Source: CAD feature listing. Evaluate the final solid. Frame: model axes, mm. A direction names the side the tool comes from. Give positions to 0.01 mm unless a question says otherwise; leave off trailing zeros. Loops run counter-clockwise (first coordinate to the right, second up) from the corner with the lowest first, then second, coordinate; pieces in that order, holes last.
```python
from build123d import *

# Parameters (mm, degrees)
SKETCH1_R               = 6.35
BOSS_EXTRUDE1_DEPTH     = 50.8
SKETCH2_W               = 82.55
SKETCH2_H               = 66.675
CUT_EXTRUDE1_DEPTH      = 20.05
CUT_EXTRUDE1_DEPTH_BACK = 20.05
FILLET1_R               = 6.35
FILLET2_R               = 9.525
FILLET3_R               = 9.525
FILLET4_R               = 9.525


with BuildPart() as part:
    # Sketch1 → Boss-Extrude1 (new body, symmetric)
    with BuildSketch(Plane(origin=(0, 0, 0), x_dir=(0, 0, -1), z_dir=(1, 0, 0))):
        with BuildLine():
            Line((9.525, 36.5125), (14.473290811, 46.0375))
            Line((14.473290811, 46.0375), (-9.525, 46.0375))
            Line((-9.525, 46.0375), (-9.525, 36.5125))
            Line((-9.525, 36.5125), (-9.525, 16.497783942))
            ThreePointArc((-9.525, 16.497783942), (-19.05, 0), (-9.525, -16.497783942))
            Line((-9.525, -16.497783942), (-9.525, -36.5125))
            Line((-9.525, -36.5125), (-14.473290811, -46.0375))
            Line((-14.473290811, -46.0375), (9.525, -46.0375))
            Line((9.525, -46.0375), (9.525, -36.5125))
            Line((9.525, -36.5125), (9.525, -16.497783942))
            ThreePointArc((9.525, -16.497783942), (19.05, 0), (9.525, 16.497783942))
            Line((9.525, 16.497783942), (9.525, 36.5125))
        make_face()
        Circle(SKETCH1_R, mode=Mode.SUBTRACT)
    extrude(amount=BOSS_EXTRUDE1_DEPTH, both=True)

    # Sketch2 → Cut-Extrude1 (cut, two sides)
    with BuildSketch(Plane.XY) as cut_extrude1_sk:
        Rectangle(SKETCH2_W, SKETCH2_H)
    extrude(amount=CUT_EXTRUDE1_DEPTH, mode=Mode.SUBTRACT)
    extrude(cut_extrude1_sk.sketch, amount=-CUT_EXTRUDE1_DEPTH_BACK, mode=Mode.SUBTRACT)

    # Fillet1
    fillet1_edges = [part.edges().sort_by_distance(p)[0] for p in [
        (-41.275, 33.3375, 0),
        (41.275, -33.3375, 0),
        (41.275, 33.3375, 0),
        (-41.275, -33.3375, 0),
    ]]
    fillet(fillet1_edges, radius=FILLET1_R)

    # Fillet2
    fillet2_edges = [part.edges().sort_by_distance(p)[0] for p in [
        (46.0375, 16.497783942, -9.525),
        (46.0375, -16.497783942, -9.525),
        (46.0375, -16.497783942, 9.525),
        (46.0375, 16.497783942, 9.525),
        (-46.0375, 16.497783942, -9.525),
        (-46.0375, -16.497783942, -9.525),
        (-46.0375, -16.497783942, 9.525),
        (-46.0375, 16.497783942, 9.525),
    ]]
    fillet(fillet2_edges, radius=FILLET2_R)

    # Fillet3
    fillet3_edges = [part.edges().sort_by_distance(p)[0] for p in [
        (0, -46.0375, -9.525),
        (0, 46.0375, 9.525),
    ]]
    fillet(fillet3_edges, radius=FILLET3_R)

    # Fillet4
    fillet4_edges = [part.edges().sort_by_distance(p)[0] for p in [
        (0, -36.5125, 9.525),
        (0, 36.5125, -9.525),
    ]]
    fillet(fillet4_edges, radius=FILLET4_R)


solid = part.part
```
(1) Ray query, line 1 along X through (y, z) = (6.5, 5) (3 decimals); line 2 along Z through (x, y) = (45, 0); line 3 along Z through (x, y) = (43, 23) (3 decimals). Return the intervals inside material, ascending.
A:
line 1: x = -50.8 to -41.275, 41.275 to 50.8
line 2: z = -19.05 to -6.35, 6.35 to 19.05
line 3: z = -9.525 to 9.525
(2) Section A-A, the plane y = 0. Return the cut outline in (x, z) (3 decimals).
A:
outline: (-50.8, -19.05) - (-41.275, -19.05) - (-41.275, -6.35) - (-50.8, -6.35) - close; (-50.8, 6.35) - (-41.275, 6.35) - (-41.275, 19.05) - (-50.8, 19.05) - close; (41.275, -19.05) - (50.8, -19.05) - (50.8, -6.35) - (41.275, -6.35) - close; (41.275, 6.35) - (50.8, 6.35) - (50.8, 19.05) - (41.275, 19.05) - close
(3) Section D-D, the plane y = -12.5. Return the cut outline in (x, z) (3 decimals), then the cut area to 3 significant figures.
A:
outline: (-50.8, -14.375) - (-41.275, -14.375) - (-41.275, 14.375) - (-50.8, 14.375) - close; (41.275, -14.375) - (50.8, -14.375) - (50.8, 14.375) - (41.275, 14.375) - close
area: 548 mm2
(4) First-contact query: pin 1 (9.5 mm diameter, centred on x = -12, z = 4.5, fed in from +Y); pin 2 (14 mm diameter, centred on x = 23.5, y = 31, fed in from -Z); pin 3 (2 mm diameter, centred on x = 18.5, y = 33.5, fed in from +Z) (3 decimals); pin 4 (12 mm diameter, centred on x = -23, y = -28, fed in from -Z) (3 decimals). Flat tips, straight axial feed; report the tip coordinate or a pass-through.
A:
pin 1: stops at y = 46.04
pin 2: stops at z = -10.32
pin 3: stops at z = 9.525
pin 4: stops at z = -9.525
(5) Reachability of faces 1 (the flat face through (1, -34, -9.525)), 2 (the cylindrical face through (-45.971, 17.461, 10.332)), 3 (the cylindrical face through (-39.365, 31.527, 0.133)), 4 (the cylindrical face through (46.104, -17.461, 10.332)), 5 (the flat face through (0.71, 42.26, -12.51)) from +Z, -Z, +X, -X, +Y, -Y: full face, straight path, thin tool, end or side. Return the list, or none.
A:
face 1: -Z, +X, -X, -Y
face 2: +Z, +X, -X, +Y
face 3: +Z, -Z
face 4: +Z, +X, -X
face 5: -Z, +X, -X
(6) Mould query, pull axis X, two halves, no side actions, for faces 6 (the flat face through (-50.8, 1, -8)), 7 (the cylindrical face through (-45.97, 0.22, 19.05)), 8 (the flat face through (0, -33.338, 0)). Classes: pulls with the +X half, pulls with the -X half, needs draft (parallel to the pull), parting line crosses it, or undercut.
A:
face 6: pulls with the -X half
face 7: needs draft
face 8: undercut
